from build123d import *

# Parameters (mm, degrees)
SKETCH1_W    = 18.6
SKETCH1_H    = 18.6
PCB_DEPTH    = 0.8
SKETCH2_W    = 18
SKETCH2_H    = 18
PATCH_DEPTH  = 4
SKETCH3_W    = 16
SKETCH3_H    = 16
RADOME_DEPTH = 2
FILLET1_R    = 2
FILLET2_R    = 0.5
SKETCH4_R    = 0.565
CABLE_DEPTH  = 12


with BuildPart() as part:
    # Sketch1 → PCB (new body)
    with BuildSketch(Plane(origin=(0, 0, 0), x_dir=(1, 0, 0), z_dir=(0, 1, 0))):
        Rectangle(SKETCH1_W, SKETCH1_H)
    extrude(amount=PCB_DEPTH)

    # Sketch2 → PATCH (add)
    with BuildSketch(Plane(origin=(0, 0.8, 0), x_dir=(1, 0, 0), z_dir=(0, 1, 0))):
        Rectangle(SKETCH2_W, SKETCH2_H)
    extrude(amount=PATCH_DEPTH)

    # Sketch3 → RADOME (add)
    with BuildSketch(Plane.XZ):
        Rectangle(SKETCH3_W, SKETCH3_H)
    extrude(amount=RADOME_DEPTH)

    # Fillet1
    fillet1_edges = [part.edges().sort_by_distance(p)[0] for p in [
        (9, 2.8, 9),
        (9, 2.8, -9),
        (-9, 2.8, -9),
        (-9, 2.8, 9),
    ]]
    fillet(fillet1_edges, radius=FILLET1_R)

    # Fillet2
    fillet2_edges = [part.edges().sort_by_distance(p)[0] for p in [
        (8, -1, -8),
        (8, -1, 8),
        (-8, -1, 8),
        (-8, -1, -8),
        (8, -2, 0),
        (0, -2, 8),
        (-8, -2, 0),
        (0, -2, -8),
    ]]
    fillet(fillet2_edges, radius=FILLET2_R)

    # Sketch4 → CABLE (add)
    with BuildSketch(Plane.XY):
        with Locations(Location((0, -0.65, 0), (0, 0, 180))):
            Circle(SKETCH4_R)
    extrude(amount=CABLE_DEPTH)


solid = part.part
Source: CAD feature listing. Evaluate the final solid. Frame: model axes, mm. A direction names the side the tool comes from. Coordinates: 2 decimals unless noted, no trailing zeros. Order: outer loops, then holes, each group sorted by start corner. A loop starts at its lowest first (then second) coordinate and runs counter-clockwise, first axis right, second up.
Item 1: First-contact query: P1, Ø2, axis at x = -6.5, y = 4, coming from the -Z side; P2, Ø2, axis at y = 3.5, z = 6, coming from the +X side; P3, Ø0.8, axis at x = -2, y = -0.5, coming from the -Z side. Flat tips, straight axial feed; report the tip coordinate or a pass-through.
Output values:
P1: stops at z = -9
P2: stops at x = 9
P3: stops at z = -8
Item 2: Cut plane B-B (z = -1.25). Return loops of the section in (x, y).
Output values:
outline: (-9.3, 0) - (-8, 0) - (-8, -1.5) arc R0.5 ccw to (-7.5, -2) - (7.5, -2) arc R0.5 ccw to (8, -1.5) - (8, 0) - (9.3, 0) - (9.3, 0.8) - (9, 0.8) - (9, 4.8) - (-9, 4.8) - (-9, 0.8) - (-9.3, 0.8) - close
Item 3: Cut plane D-D (y = -0.65). Return loops of the section in (x, z) (3 decimals).
Output values:
outline: (-8, -7.5) arc R0.5 ccw to (-7.5, -8) - (7.5, -8) arc R0.5 ccw to (8, -7.5) - (8, 7.5) arc R0.5 ccw to (7.5, 8) - (0.565, 8) - (0.565, 12) - (-0.565, 12) - (-0.565, 8) - (-7.5, 8) arc R0.5 ccw to (-8, 7.5) - close
Item 4: Cut plane A-A (z = 8.5). Return loops of the section in (x, y) (3 decimals).
Output values:
outline: (-9.3, 0) - (9.3, 0) - (9.3, 0.8) - (8.323, 0.8) - (8.323, 4.8) - (-8.323, 4.8) - (-8.323, 0.8) - (-9.3, 0.8) - close; circle Ø1.13 at (0, -0.65)
Item 5: Set-up query: faces 1 (the face through (-8.4, 2.83, 8.43)), 2 (the face through (8, -1, 0)), 3 (the face through (-9, 3, 0)), 4 (the face through (8.43, 2.83, -8.4)). Return all of +Z, -Z, +X, -X, +Y, -Y with unobstructed straight access to the full face (end or side cutting, diameter ignored); none if empty.
Output values:
face 1: +Z, -X, +Y
face 2: +Z, -Z, +X, -Y
face 3: +Z, -Z, -X, +Y
face 4: -Z, +X, +Y
Item 6: Cut plane C-C (x = -4.5). Return loops of the section in (y, z), plus the area to 3 significant figures.
Output values:
outline: (-2, -7.5) arc R0.5 ccw to (-1.5, -8) - (0, -8) - (0, -9.3) - (0.8, -9.3) - (0.8, -9) - (4.8, -9) - (4.8, 9) - (0.8, 9) - (0.8, 9.3) - (0, 9.3) - (0, 8) - (-1.5, 8) arc R0.5 ccw to (-2, 7.5) - close
area: 119 mm2
Item 7: Material intervals for line 1 (Z direction, x = -1.75, y = 2.75); line 2 (Y direction, x = -4.75, z = 9.25), sorted ascending.
Output values:
line 1: z = -9 to 9
line 2: y = 0 to 0.8
